Here's how the part is built. I have some questions about the finished solid (model axes, mm). Face numbers are marked on the shaded views. A direction names the side the tool comes from. Round coordinates to 2 decimals unless told otherwise and drop trailing zeros. Loops run counter-clockwise (first coordinate to the right, second up) from the corner with the lowest first, then second, coordinate; pieces in that order, holes last. Notation, with made-up numbers: M 4,-24.5 L 51,-24.5 A24 cw 51,-10.5 Z; hole C 87.5,67.5 d10. An arc over 180 degrees is marked long. Answer as a JSON object with one key per item and string values.
from build123d import *

# Parameters (mm, degrees)
BOSS_EXTRUDE1_DEPTH = 2.5
SKETCH5_W           = 2.85
SKETCH5_H           = 2.5
CUT_EXTRUDE2_DEPTH  = 7.5
SKETCH6_W           = 2.85
SKETCH6_H           = 2.5
CUT_EXTRUDE3_DEPTH  = 7.5
SKETCH7_W           = 2.85
SKETCH7_H           = 2.5
CUT_EXTRUDE4_DEPTH  = 7.5


with BuildPart() as part:
    # Sketch1 → Boss-Extrude1 (new body)
    with BuildSketch(Plane(origin=(0, 0, 0), x_dir=(1, 0, 0), z_dir=(0, 1, 0))):
        Polygon((8.581310361, -0.009375041), (4.251183342, 7.490624959), (-8.409070695, 7.490624959), (-12.739197714, -0.009375041), (-8.409070695, -7.509375041), (4.251183342, -7.509375041), align=None)
    extrude(amount=BOSS_EXTRUDE1_DEPTH)

    # Sketch5 → Cut-Extrude2 (cut)
    with BuildSketch(Plane.XY.offset(7.509375041)):
        with Locations((-6.984070695, 1.25)):
            Rectangle(SKETCH5_W, SKETCH5_H)
    extrude(amount=-CUT_EXTRUDE2_DEPTH, mode=Mode.SUBTRACT)

    # Sketch6 → Cut-Extrude3 (cut)
    with BuildSketch(Plane.XY.offset(7.509375041)):
        with Locations((2.826183342, 1.25)):
            Rectangle(SKETCH6_W, SKETCH6_H)
    extrude(amount=-CUT_EXTRUDE3_DEPTH, mode=Mode.SUBTRACT)

    # Sketch7 → Cut-Extrude4 (cut)
    with BuildSketch(Plane(origin=(0, 0, -7.490624959), x_dir=(-1, 0, 0), z_dir=(0, 0, -1))):
        with Locations((2.083816658, 1.25)):
            Rectangle(SKETCH7_W, SKETCH7_H)
    extrude(amount=-CUT_EXTRUDE4_DEPTH, mode=Mode.SUBTRACT)


solid = part.part
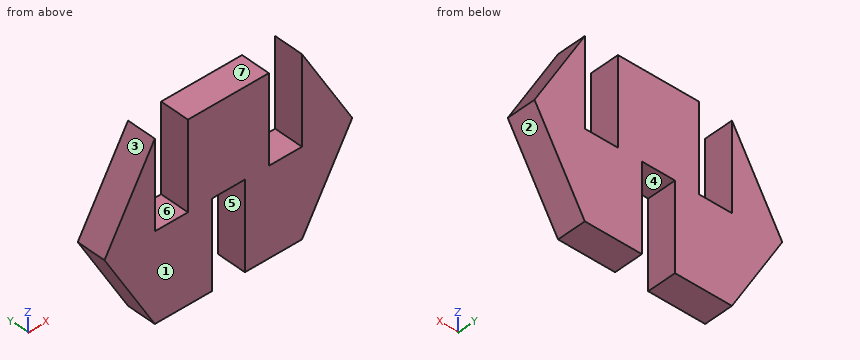
Item 1: For the marked faces 5, 6 and 7, which set-ups out of +Z, -Z, +X, -X, +Y, -Y let a thin tool reach every point of the face, with its end or its side?
Solution:
{"face 5": "-Z, +Y, -Y", "face 6": "+Z, +Y, -Y", "face 7": "+Z, +X, -X, +Y, -Y"}
Item 2: I want a section at C-C on z = 4.5. List the corners of the cut face in (x, y) for me.
Solution:
{"outline": "M -10.15,0 L -8.41,0 L -8.41,2.5 L -10.15,2.5 Z; M -5.56,0 L 1.4,0 L 1.4,2.5 L -5.56,2.5 Z; M 4.25,0 L 5.99,0 L 5.99,2.5 L 4.25,2.5 Z"}
Item 3: If I drill on L1, parallel to X at y = 1, z = 5; L2, parallel to X at y = 1.75, z = 4.75; L3, parallel to X at y = 2.1, z = -4.75, over which ranges is the centre line in solid material (lowest first)? Write a range as from..to.
Solution:
{"L1": "x = -9.86..-8.41, -5.56..1.4, 4.25..5.7", "L2": "x = -10..-8.41, -5.56..1.4, 4.25..5.84", "L3": "x = -9.99..-3.51, -0.66..5.83"}
Item 4: For P1, Ø0.8, axis at x = -2.5, y = 1, coming from the -Z side; P2, Ø1.5, axis at y = 2, z = 5.5, coming from the -X side; P3, Ø0.8, axis at y = 1, z = 2, coming from the -X side; P4, Ø4, axis at x = 2, z = 4, coming from the -Y side, each with a flat end and sliding along its axis, tell me the tip position at first contact or that it passes through.
Solution:
{"P1": "stops at z = 0.01", "P2": "stops at x = -10", "P3": "stops at x = -11.82", "P4": "stops at y = 0"}
Item 5: I want a section at D-D on x = -2.25. List the corners of the cut face in (y, z) for me, plus the area to 4 significant figures.
Solution:
{"outline": "M 0,0.01 L 2.5,0.01 L 2.5,7.51 L 0,7.51 Z", "area": "18.75 mm2"}
Item 6: We'd pull the mould along X, two halves only. Please class the marked faces 1, 2, 3 and 4: +X half, -X half, draft (parallel to the pull), parting line (faces both ways), or undercut.
Solution:
{"face 1": "draft", "face 2": "+X half", "face 3": "-X half", "face 4": "undercut"}
Item 7: I want a section at A-A on z = -1.25. List the corners of the cut face in (x, y) for me.
Solution:
{"outline": "M -12.01,0 L -3.51,0 L -3.51,2.5 L -12.01,2.5 Z; M -0.66,0 L 7.85,0 L 7.85,2.5 L -0.66,2.5 Z"}
Item 8: I want a section at B-B on y = 1.15. List the corners of the cut face in (x, z) for me.
Solution:
{"outline": "M -12.74,0.01 L -8.41,-7.49 L -3.51,-7.49 L -3.51,0.01 L -0.66,0.01 L -0.66,-7.49 L 4.25,-7.49 L 8.58,0.01 L 4.25,7.51 L 4.25,0.01 L 1.4,0.01 L 1.4,7.51 L -5.56,7.51 L -5.56,0.01 L -8.41,0.01 L -8.41,7.51 Z"}
